Input: part model. Units: mm. Frame: model coordinates. Coordinates: 2 decimals unless noted, no trailing zeros. Loops run counter-clockwise (first coordinate to the right, second up) from the corner with the lowest first, then second, coordinate; pieces in that order, holes last. Notation, with made-up numbers: (52.5, -16.5) -> (60.5, -16.5) arc R25 ccw to (60.5, 7.5) -> close; hole circle Ø7 at (82.25, 58.25). An arc over 180 degrees is marked (long way). Put each result on its own line as item: value. Start each with the question number.
1) Cut plane B-B (y = 1.3). Return the cut outline in (x, z), plus the area to 3 significant figures.
2) Cut plane A-A (x = 23.5). Return the cut outline in (y, z), plus the area to 3 significant figures.
3) Contact query for flat-ended pins moving along their axis: P1, Ø2, axis at x = -17.5, y = -1.5, coming from the +Z side; P2, Ø1, axis at x = 24.5, y = -1, coming from the -Z side; P3, Ø2.5, axis at x = 24, z = -12.5, coming from the +Y side; P4, Ø1.5, axis at x = 23.5, z = 14.5, coming from the +Y side. Output: stop coordinate, or through.
4) Material intervals for L1, parallel to Z at x = 6.5, y = -0.7; L2, parallel to Z at x = 23, y = 1.35; L3, parallel to X at y = 0.95, z = -3, sorted ascending.
from build123d import *

# Parameters (mm, degrees)
SKETCH1_W           = 52
SKETCH1_H           = 37
BOSS_EXTRUDE1_DEPTH = 1.9
SKETCH2_W           = 5
SKETCH2_H           = 9
CUT_EXTRUDE1_DEPTH  = 1.25
CUT_EXTRUDE2_DEPTH  = 3.55
CHAMFER1_SIZE       = 1.5
FILLET2_R           = 1.5


with BuildPart() as part:
    # Sketch1 → Boss-Extrude1 (new body, symmetric)
    with BuildSketch(Plane(origin=(0, 0, 0), x_dir=(1, 0, 0), z_dir=(0, 1, 0))):
        Rectangle(SKETCH1_W, SKETCH1_H)
    extrude(amount=BOSS_EXTRUDE1_DEPTH, both=True)

    # Sketch2 → Cut-Extrude1 (cut)
    with BuildSketch(Plane(origin=(0, 1.9, 0), x_dir=(1, 0, 0), z_dir=(0, 1, 0))):
        with Locations((23.5, 14)):
            Rectangle(SKETCH2_W, SKETCH2_H)
        with Locations((23.5, -14)):
            Rectangle(SKETCH2_W, SKETCH2_H)
    cut_extrude1 = extrude(amount=-CUT_EXTRUDE1_DEPTH, mode=Mode.SUBTRACT)

    # Mirror1: Cut-Extrude1 across plane
    add(cut_extrude1.mirror(Plane.ZX), mode=Mode.SUBTRACT)

    # Sketch3 → Cut-Extrude2 (cut, through all)
    with BuildSketch(Plane(origin=(0, 0.65, 0), x_dir=(1, 0, 0), z_dir=(0, 1, 0))):
        with BuildLine():
            Line((22.5, 12), (22.5, 16))
            ThreePointArc((22.5, 16), (23.5, 17), (24.5, 16))
            Line((24.5, 16), (24.5, 12))
            ThreePointArc((24.5, 12), (23.5, 11), (22.5, 12))
        make_face()
        with BuildLine():
            Line((22.5, -12), (22.5, -16))
            ThreePointArc((22.5, -16), (23.5, -17), (24.5, -16))
            Line((24.5, -16), (24.5, -12))
            ThreePointArc((24.5, -12), (23.5, -11), (22.5, -12))
        make_face()
    extrude(amount=-CUT_EXTRUDE2_DEPTH, mode=Mode.SUBTRACT)

    # Chamfer1
    chamfer1_edges = [part.edges().sort_by_distance(p)[0] for p in [
        (26, 0, -18.5),
        (26, 0, 18.5),
    ]]
    chamfer(chamfer1_edges, length=CHAMFER1_SIZE)

    # Fillet2
    fillet2_edges = [part.edges().sort_by_distance(p)[0] for p in [
        (-2.5, -1.9, -18.5),
        (-26, 0, -18.5),
        (-26, 0, 18.5),
        (-26, -1.9, 0),
        (-2.5, -1.9, 18.5),
        (-2.5, 1.9, 18.5),
        (-26, 1.9, 0),
        (-2.5, 1.9, -18.5),
    ]]
    fillet(fillet2_edges, radius=FILLET2_R)


solid = part.part
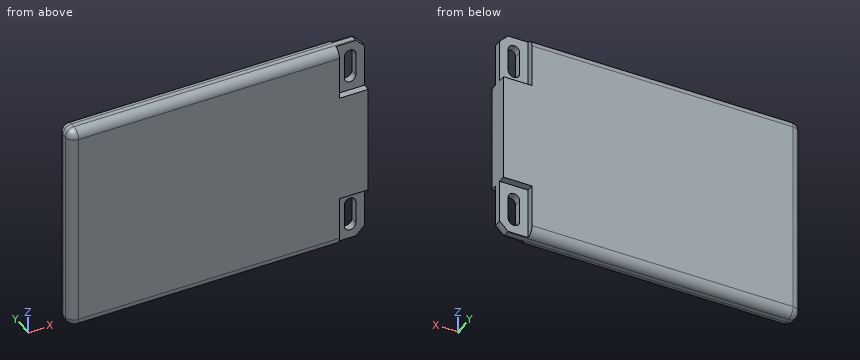
Results found:
1. outline: (-25.7, -17) arc R1.2 ccw to (-24.5, -18.2) -> (21, -18.2) -> (21, -9.5) -> (26, -9.5) -> (26, 9.5) -> (21, 9.5) -> (21, 18.2) -> (-24.5, 18.2) arc R1.2 ccw to (-25.7, 17) -> close
1. area: 1,790 mm2
2. outline: (-1.9, -9.5) -> (-0.65, -9.5) -> (-0.65, -11) -> (0.65, -11) -> (0.65, -9.5) -> (1.9, -9.5) -> (1.9, 9.5) -> (0.65, 9.5) -> (0.65, 11) -> (-0.65, 11) -> (-0.65, 9.5) -> (-1.9, 9.5) -> close; (-0.65, -18.48) arc R1.5 ccw to (-0.4, -18.5) -> (0.4, -18.5) arc R1.5 ccw to (0.65, -18.48) -> (0.65, -17) -> (-0.65, -17) -> close; (-0.65, 17) -> (0.65, 17) -> (0.65, 18.48) arc R1.5 ccw to (0.4, 18.5) -> (-0.4, 18.5) arc R1.5 ccw to (-0.65, 18.48) -> close
2. area: 80.0 mm2
3. P1: stops at z = 18.5
3. P2: stops at z = -18.5
3. P3: stops at y = 0.65
3. P4: passes through
4. L1: z = -18.47 to 18.47
4. L2: z = -9.5 to 9.5
4. L3: x = -25.9 to 26
